Could you check a few things on this model? Use its own coordinates, in mm. A direction names the side the tool comes from. Give positions to 0.01 mm unless a question says otherwise; leave off trailing zeros. Write each loop counter-clockwise with the first axis right and the second up, starting at its lowest first coordinate (ties: lowest second). Pieces come first, ordered by that corner, then holes. Notation, with made-up numbers: M 63,85 L 71,85 A21 ccw 71,111 Z; hole C 54,81.5 d10. An arc over 180 degrees is marked long. Use one line per item in the form item = value.
from build123d import *

# Parameters (mm, degrees)
SKETCH1_R                    = 76.2
BOSS_EXTRUDE1_DEPTH          = 30
CIRPATTERN1_COUNT            = 3
F_10_0_1935_DIAMETER_HOLE1_D = 4.9149
CIRPATTERN2_COUNT            = 12
CIRPATTERN3_COUNT            = 6
SKETCH21_W                   = 5
SKETCH21_H                   = 3
CIRPATTERN4_COUNT            = 6
SKETCH29_R                   = 55.14
SKETCH29_R_2                 = 5.953252
BOSS_EXTRUDE2_DEPTH          = 2


with BuildPart() as part:
    # Sketch1 → Boss-Extrude1 (new body)
    with BuildSketch(Plane(origin=(0, 0, 0), x_dir=(1, 0, 0), z_dir=(0, 1, 0))):
        with Locations(Location((0, 0, 0), (0, 0, 270))):
            Circle(SKETCH1_R)
    extrude(amount=BOSS_EXTRUDE1_DEPTH)

    # Sketch2 → Cut-Revolve1 (revolve, cut)
    with BuildSketch(Plane.XY):
        with BuildLine():
            Line((-5.953252, 0), (-5.953252, 4.113248654))
            ThreePointArc((-5.953252, 4.113248654), (-6.623124981, 6.613248654), (-8.453252, 8.443375673))
            Line((-8.453252, 8.443375673), (-13.5, 11.357116989))
            ThreePointArc((-13.5, 11.357116989), (-15.330127019, 13.187244008), (-16, 15.687244008))
            Line((-16, 15.687244008), (-16, 30))
            Line((-16, 30), (0, 30))
            Line((0, 30), (0, 0))
            Line((0, 0), (-5.953252, 0))
        make_face()
    revolve(axis=Axis((0, 30, 0), (0, -1, 0)), mode=Mode.SUBTRACT)

    # Sketch5 → 1/4 NPT Tapped Hole1 (revolve, cut)
    with BuildSketch(Plane(origin=(0, 18.904757199, 80.54), x_dir=(0, -1, 0), z_dir=(1, 0, 0))):
        Polygon((0, 0), (0, 83.882347279), (5.5626, 80.54), (5.5626, 10.02), (6.58554395, 10.02), (6.8579873, 0.9207627), (7.77875, 0), align=None)
    f_1_4_npt_tapped_hole1 = revolve(axis=Axis((0, 18.904757199, 86.89), (0, 0, -1)), mode=Mode.SUBTRACT)

    # CirPattern1: 1/4 NPT Tapped Hole1 ×3 about axis
    cirpattern1_axis = Axis((0, 0, 0), (0, 1, 0))
    for i in range(1, CIRPATTERN1_COUNT):
        add(f_1_4_npt_tapped_hole1.rotate(cirpattern1_axis, i * 360 / CIRPATTERN1_COUNT), mode=Mode.SUBTRACT)

    # #10 (0.1935) Diameter Hole1 (through all)
    with Locations(Plane(origin=(0, 30, 0), x_dir=(1, 0, 0), z_dir=(0, 1, 0))):
        with Locations((-17.814475001, 66.660666667)):
            f_10_0_1935_diameter_hole1 = Hole(F_10_0_1935_DIAMETER_HOLE1_D / 2)

    # CirPattern2: #10 (0.1935) Diameter Hole1 ×12 about axis
    cirpattern2_axis = Axis((0, 0, 0), (0, 1, 0))
    for i in range(1, CIRPATTERN2_COUNT):
        add(f_10_0_1935_diameter_hole1.rotate(cirpattern2_axis, i * 360 / CIRPATTERN2_COUNT), mode=Mode.SUBTRACT)

    # Sketch19 → 13/64 (0.20313) Diameter Hole3 (revolve, cut)
    with BuildSketch(Plane(origin=(30.305, 30, -52.489799723), x_dir=(0, 0, 1), z_dir=(1, 0, 0))):
        Polygon((0, 0), (0, 14.250070783), (2.579751, 12.7), (2.579751, 0), align=None)
    f_13_64_0_20313_diameter_hole3 = revolve(axis=Axis((30.305, 36.35, -52.489799723), (0, -1, 0)), mode=Mode.SUBTRACT)

    # CirPattern3: 13/64 (0.20313) Diameter Hole3 ×6 about axis
    cirpattern3_axis = Axis((0, 0, 0), (0, 1, 0))
    for i in range(1, CIRPATTERN3_COUNT):
        add(f_13_64_0_20313_diameter_hole3.rotate(cirpattern3_axis, i * 360 / CIRPATTERN3_COUNT), mode=Mode.SUBTRACT)

    # Sketch21 → Cut-Revolve2 (revolve, cut)
    with BuildSketch(Plane.XY, mode=Mode.PRIVATE) as cut_revolve2_sk:
        with Locations((62.5, 1.5)):
            Rectangle(SKETCH21_W, SKETCH21_H)
    revolve(cut_revolve2_sk.sketch.rotate(Axis((0, 0, 0), (0, -1, 0)), 90), axis=Axis((0, 0, 0), (0, -1, 0)), mode=Mode.SUBTRACT)

    # Sketch28 → 3/16 (0.1875) Diameter Hole1 (revolve, cut)
    with BuildSketch(Plane(origin=(29, 30, 0), x_dir=(0, 0, 1), z_dir=(1, 0, 0))):
        Polygon((0, 0), (0, 13.430799349), (2.38125, 12), (2.38125, 0), align=None)
    f_3_16_0_1875_diameter_hole1 = revolve(axis=Axis((29, 36.35, 0), (0, -1, 0)), mode=Mode.SUBTRACT)

    # CirPattern4: 3/16 (0.1875) Diameter Hole1 ×6 about axis
    cirpattern4_axis = Axis((0, 0, 0), (0, 1, 0))
    for i in range(1, CIRPATTERN4_COUNT):
        add(f_3_16_0_1875_diameter_hole1.rotate(cirpattern4_axis, i * 360 / CIRPATTERN4_COUNT), mode=Mode.SUBTRACT)

    # Sketch29 → Boss-Extrude2 (add)
    with BuildSketch(Plane(origin=(0, 0, 0), x_dir=(-1, 0, 0), z_dir=(0, -1, 0))):
        with Locations(Location((0, 0, 0), (0, 0, 90))):
            Circle(SKETCH29_R)
        Circle(SKETCH29_R_2, mode=Mode.SUBTRACT)
    extrude(amount=BOSS_EXTRUDE2_DEPTH)


solid = part.part
1) If I drill on L1, parallel to X at y = 1, z = 44; L2, parallel to X at y = 0.5, z = -46; L3, parallel to X at y = 24.5, z = 8.5, over which ranges is the centre line in solid material (lowest first)?
Checked values:
L1 = -62.21 to -47.84, -40.79 to 40.79, 47.84 to 62.21
L2 = -60.75 to -45.92, -38.52 to 38.52, 45.92 to 60.75
L3 = -75.72 to -13.56, 13.56 to 75.72
2) I want a section at B-B, the plane y = 22.5. Count the separate pieces of the cut face and the enclosed holes in it, plus the area to 3 significant figures.
Checked values:
separate_pieces = 3
enclosed_holes = 24
area = 15,400 mm2
3) For faces 4 (the cylindrical face through (64.293, 14.79, 17.164)), 5 (the cylindrical face through (15.215, 24.084, 22.843)), 6 (the flat face through (62, 0, 22)), which set-ups out of +Z, -Z, +X, -X, +Y, -Y let a thin tool reach every point of the face, with its end or its side?
Checked values:
face_4 = +Y, -Y
face_5 = +Y
face_6 = -Y
4) For pin 1 Ø4 at (y, z) = (9, -56) entering from -X; pin 2 Ø4 at (x, y) = (12, 11.5) entering from -Z; pin 3 Ø15.5 at (x, z) = (0, 0) entering from +Y, each with a flat end and sliding along its axis, tell me the tip position at first contact or that it passes through.
Checked values:
pin_1 = -53.76
pin_2 = -75.54
pin_3 = 7.95
5) Thinking about a two-plate mould opening in Z: for faces 1 (the cylindrical face through (17.164, 14.79, -64.293)), 2 (the flat face through (63.527, 15.947, -31.009)), 3 (the flat face through (-11, -2, 1)), which applies, released by +Z, released by -Z, zero draft, split by the parting line, or undercut?
Checked values:
face_1 = undercut
face_2 = undercut
face_3 = zero draft
6) I want a section at A-A, the plane z = 36. Please give me the cut outline in (x, y).
Checked values:
outline = M -67.16,0 L -54.12,0 L -54.12,3 L -48,3 L -48,0 L -41.77,0 L -41.77,-2 L 41.77,-2 L 41.77,0 L 48,0 L 48,3 L 54.12,3 L 54.12,0 L 67.16,0 L 67.16,30 L -67.16,30 Z; hole C 0,18.9 d11.13
